Could you check a few things on this drawing? It's one solid part, dimensions in mm from its lowest x, y, z. A direction names the side the tool comes from. Round coordinates to 2 decimals unless told otherwise and drop trailing zeros. Loops run counter-clockwise (first coordinate to the right, second up) from the corner with the lowest first, then second, coordinate; pieces in that order, holes last.
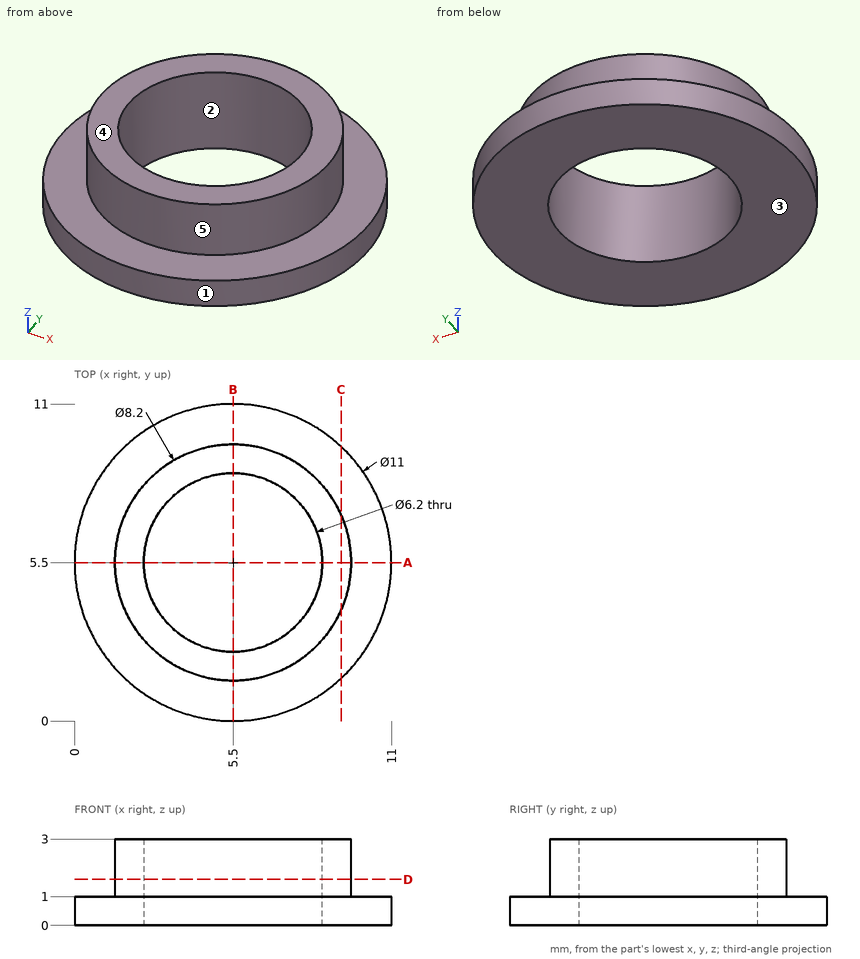
(1) Suppose I cut it at D-D (z = 1.6). Write out the boundary of the cut face in (x, y).
(2) Suppose I cut it at A-A (y = 5.5). Write out the boundary of the cut face in (x, z).
(3) We'd pull the mould along Y, two halves only. Please class the marked faces 1, 2 and 3: released by +Y, released by -Y, zero draft, split by the parting line, or undercut.
(4) Suppose I cut it at C-C (x = 9.25). Write out the boundary of the cut face in (y, z).
(5) For pin 1 (1.5 mm diameter, centred on x = 2, z = 2, fed in from +Y); pin 2 (5.5 mm diameter, centred on x = 5.5, y = 7, fed in from +Z), each with a flat end and sliding along its axis, tell me the tip position at first contact or that it passes through.
(6) Which directions (+Z, -Z, +X, -X, +Y, -Y) give clear straight access to the entire face, cutting with the end or side of a thin tool? Please do the marked faces 4 and 5.
(7) If I drill on line 1 (X direction, y = 5.5, z = 1.9); line 2 (Z direction, x = 1.5, y = 2.75), over which ranges is the centre line in solid material (lowest first)?
Check result:
1. outline: circle Ø8.2 at (5.5, 5.5); hole circle Ø6.2 at (5.5, 5.5)
2. outline: (0, 0) - (2.4, 0) - (2.4, 3) - (1.4, 3) - (1.4, 1) - (0, 1) - close; (8.6, 0) - (11, 0) - (11, 1) - (9.6, 1) - (9.6, 3) - (8.6, 3) - close
3. face 1: split by the parting line
3. face 2: undercut
3. face 3: zero draft
4. outline: (1.48, 0) - (9.52, 0) - (9.52, 1) - (7.16, 1) - (7.16, 3) - (3.84, 3) - (3.84, 1) - (1.48, 1) - close
5. pin 1: stops at y = 8.54
5. pin 2: stops at z = 3
6. face 4: +Z, +X, -X, +Y, -Y
6. face 5: +Z
7. line 1: x = 1.4 to 2.4, 8.6 to 9.6
7. line 2: z = 0 to 1
